```python
from build123d import *

# Parameters (mm, degrees)
SKETCH1_R           = 25
SKETCH1_R_2         = 2.5
BOSS_EXTRUDE1_DEPTH = 5
SKETCH2_R           = 16
CUT_EXTRUDE1_DEPTH  = 36.707142143
SKETCH3_R           = 5
SKETCH3_R_2         = 2.5
BOSS_EXTRUDE2_DEPTH = 5
BOSS_EXTRUDE3_START = 35
SKETCH4_R           = 15
SKETCH4_R_2         = 2.5
BOSS_EXTRUDE3_DEPTH = 35
CUT_EXTRUDE2_START  = -19
SKETCH5_R           = 15
CUT_EXTRUDE2_DEPTH  = 14


with BuildPart() as part:
    # Sketch1 → Boss-Extrude1 (new body)
    with BuildSketch(Plane(origin=(0, 0, 0), x_dir=(1, 0, 0), z_dir=(0, 1, 0))):
        with Locations(Location((0, 0, 0), (0, 0, 270))):
            Circle(SKETCH1_R)
        with Locations(Location((0, 0, 0), (0, 0, 270))):
            Circle(SKETCH1_R_2, mode=Mode.SUBTRACT)
    extrude(amount=BOSS_EXTRUDE1_DEPTH)

    # Sketch2 → Cut-Extrude1 (cut, through all)
    with BuildSketch(Plane(origin=(0, 5, 0), x_dir=(1, 0, 0), z_dir=(0, 1, 0))):
        with Locations((22.627416998, 22.627416998)):
            Circle(SKETCH2_R)
        with Locations((-22.627416998, 22.627416998)):
            Circle(SKETCH2_R)
        with BuildLine():
            Line((-2.5, 24.874685928), (-2.5, 7.5))
            ThreePointArc((-2.5, 7.5), (0, 5), (2.5, 7.5))
            Line((2.5, 7.5), (2.5, 24.874685928))
            ThreePointArc((2.5, 24.874685928), (0, 25), (-2.5, 24.874685928))
        make_face()
    extrude(amount=-CUT_EXTRUDE1_DEPTH, mode=Mode.SUBTRACT)

    # Sketch3 → Boss-Extrude2 (add)
    with BuildSketch(Plane(origin=(0, 5, 0), x_dir=(1, 0, 0), z_dir=(0, 1, 0))):
        with Locations(Location((0, 0, 0), (0, 0, 90))):
            Circle(SKETCH3_R)
        with Locations(Location((0, 0, 0), (0, 0, 270))):
            Circle(SKETCH3_R_2, mode=Mode.SUBTRACT)
    extrude(amount=BOSS_EXTRUDE2_DEPTH)

    # Sketch4 → Boss-Extrude3 (add)
    with BuildSketch(Plane.XZ.offset(BOSS_EXTRUDE3_START)):
        with Locations(Location((0, 0, 0), (0, 0, 260.405931773))):
            Circle(SKETCH4_R)
        with Locations(Location((0, 0, 0), (0, 0, 270))):
            Circle(SKETCH4_R_2, mode=Mode.SUBTRACT)
    extrude(amount=-BOSS_EXTRUDE3_DEPTH)

    # Sketch5 → Cut-Extrude2 (cut)
    with BuildSketch(Plane(origin=(0, 0, 0), x_dir=(1, 0, 0), z_dir=(0, 1, 0)).offset(CUT_EXTRUDE2_START)):
        with Locations(Location((0, 0, 0), (0, 0, 270))):
            Circle(SKETCH5_R)
        with BuildLine():
            Line((-10.5, 1.5), (-10.5, -1.5))
            Line((-10.5, -1.5), (-12.245822961, -2.507951357))
            ThreePointArc((-12.245822961, -2.507951357), (-11.888206454, -3.86271243), (-11.381215706, -5.16893887))
            Line((-11.381215706, -5.16893887), (-9.376356319, -4.958219658))
            Line((-9.376356319, -4.958219658), (-7.613000562, -7.385270641))
            Line((-7.613000562, -7.385270641), (-8.432942065, -9.226889407))
            ThreePointArc((-8.432942065, -9.226889407), (-7.347315654, -10.11271243), (-6.169370885, -10.871470134))
            Line((-6.169370885, -10.871470134), (-4.671263215, -9.52256793))
            Line((-4.671263215, -9.52256793), (-1.818093666, -10.449618913))
            Line((-1.818093666, -10.449618913), (-1.398963925, -12.421469315))
            ThreePointArc((-1.398963925, -12.421469315), (0, -12.5), (1.398963925, -12.421469315))
            Line((1.398963925, -12.421469315), (1.818093666, -10.449618913))
            Line((1.818093666, -10.449618913), (4.671263215, -9.52256793))
            Line((4.671263215, -9.52256793), (6.169370885, -10.871470134))
            ThreePointArc((6.169370885, -10.871470134), (7.347315654, -10.11271243), (8.432942065, -9.226889407))
            Line((8.432942065, -9.226889407), (7.613000562, -7.385270641))
            Line((7.613000562, -7.385270641), (9.376356319, -4.958219658))
            Line((9.376356319, -4.958219658), (11.381215706, -5.16893887))
            ThreePointArc((11.381215706, -5.16893887), (11.888206454, -3.86271243), (12.245822961, -2.507951357))
            Line((12.245822961, -2.507951357), (10.5, -1.5))
            Line((10.5, -1.5), (10.5, 1.5))
            Line((10.5, 1.5), (12.245822961, 2.507951357))
            ThreePointArc((12.245822961, 2.507951357), (11.888206454, 3.86271243), (11.381215706, 5.16893887))
            Line((11.381215706, 5.16893887), (9.376356319, 4.958219658))
            Line((9.376356319, 4.958219658), (7.613000562, 7.385270641))
            Line((7.613000562, 7.385270641), (8.432942065, 9.226889407))
            ThreePointArc((8.432942065, 9.226889407), (7.347315654, 10.11271243), (6.169370885, 10.871470134))
            Line((6.169370885, 10.871470134), (4.671263215, 9.52256793))
            Line((4.671263215, 9.52256793), (1.818093666, 10.449618913))
            Line((1.818093666, 10.449618913), (1.398963925, 12.421469315))
            ThreePointArc((1.398963925, 12.421469315), (0, 12.5), (-1.398963925, 12.421469315))
            Line((-1.398963925, 12.421469315), (-1.818093666, 10.449618913))
            Line((-1.818093666, 10.449618913), (-4.671263215, 9.52256793))
            Line((-4.671263215, 9.52256793), (-6.169370885, 10.871470134))
            ThreePointArc((-6.169370885, 10.871470134), (-7.347315654, 10.11271243), (-8.432942065, 9.226889407))
            Line((-8.432942065, 9.226889407), (-7.613000562, 7.385270641))
            Line((-7.613000562, 7.385270641), (-9.376356319, 4.958219658))
            Line((-9.376356319, 4.958219658), (-11.381215706, 5.16893887))
            ThreePointArc((-11.381215706, 5.16893887), (-11.888206454, 3.86271243), (-12.245822961, 2.507951357))
            Line((-12.245822961, 2.507951357), (-10.5, 1.5))
        make_face(mode=Mode.SUBTRACT)
    extrude(amount=CUT_EXTRUDE2_DEPTH, mode=Mode.SUBTRACT)


solid = part.part
```
Can you work these out from the model? Positions are in its coordinate system, mm. A direction names the side the tool comes from. Coordinates: 2 decimals unless noted, no trailing zeros. Loops run counter-clockwise (first coordinate to the right, second up) from the corner with the lowest first, then second, coordinate; pieces in that order, holes last. Notation, with made-up numbers: (56.25, 44) -> (105.25, 44) arc R19 cw to (105.25, 77) -> close; hole circle Ø4 at (17.5, 77). An arc over 180 degrees is marked (long way). Answer as a JSON object with one key per item and string values.
1) Imagine slicing it at C-C (z = -22). Please give me the cut outline in (x, y).
Results:
{"outline": "(-6.64, 0) -> (-2.5, 0) -> (-2.5, 5) -> (-6.64, 5) -> close; (2.5, 0) -> (6.64, 0) -> (6.64, 5) -> (2.5, 5) -> close"}
2) Imagine slicing it at D-D (y = -1). Please give me the cut outline in (x, z).
Results:
{"outline": "circle Ø30 at (0, 0); hole circle Ø5 at (0, 0)"}
3) If I drill on line 1 (Y direction, x = -2, z = -12); line 2 (X direction, y = -25.5, z = 0); line 3 (Y direction, x = -10, z = -8), over which ranges is the centre line in solid material (lowest first)?
Results:
{"line 1": "y = -35 to -19, -5 to 0", "line 2": "x = -15 to -2.5, 2.5 to 15", "line 3": "y = -35 to -19, -5 to 5"}
4) Imagine slicing it at B-B (x = 14). Please give me the cut outline in (y, z).
Results:
{"outline": "(-35, -5.39) -> (-19, -5.39) -> (-19, 5.39) -> (-35, 5.39) -> close; (-5, -5.39) -> (0, -5.39) -> (0, -9.15) -> (5, -9.15) -> (5, 20.71) -> (0, 20.71) -> (0, 5.39) -> (-5, 5.39) -> close"}
5) Imagine slicing it at A-A (z = 0). Please give me the cut outline in (x, y), then the cut area to 3 significant figures.
Results:
{"outline": "(-25, 0) -> (-15, 0) -> (-15, -5) -> (-10.5, -5) -> (-10.5, -19) -> (-15, -19) -> (-15, -35) -> (-2.5, -35) -> (-2.5, 10) -> (-5, 10) -> (-5, 5) -> (-25, 5) -> close; (2.5, -35) -> (15, -35) -> (15, -19) -> (10.5, -19) -> (10.5, -5) -> (15, -5) -> (15, 0) -> (25, 0) -> (25, 5) -> (5, 5) -> (5, 10) -> (2.5, 10) -> close", "area": "999 mm^2"}
6) Thinking about a two-plate mould opening in Y: for faces 1 (the face through (1.61, -12.1, -11.42)), 2 (the face through (-11.45, 2.54, -11.18)), which applies, pulls with the +Y half, pulls with the -Y half, needs draft (parallel to the pull), parting line crosses it, or undercut?
Results:
{"face 1": "undercut", "face 2": "needs draft"}
7) For P1, Ø10, axis at y = -3, z = 7.5, coming from the +X side; P2, Ø4, axis at y = 3.5, z = -18, coming from the +X side; P3, Ø10, axis at x = 17.5, z = 4.5, coming from the -Y side; P4, Ø1.5, axis at y = 3.5, z = -13, coming from the -X side, each with a flat end and sliding along its axis, tell me the tip position at first contact or that it passes through.
Results:
{"P1": "stops at x = 24.75", "P2": "stops at x = 8.06", "P3": "stops at y = -35", "P4": "stops at x = -10.45"}
8) For faces 3 (the face through (-1.61, -12.1, 11.42)), 4 (the face through (-7.331, -12.098, -10.124)), 5 (the face through (-8.017, -12.098, 8.293)), 6 (the face through (-3.2, -12.1, -10)), which set-ups out of +Z, -Z, +X, -X, +Y, -Y let a thin tool reach every point of the face, with its end or its side?
Results:
{"face 3": "+Z", "face 4": "-Z, -X", "face 5": "-X", "face 6": "-Z"}
